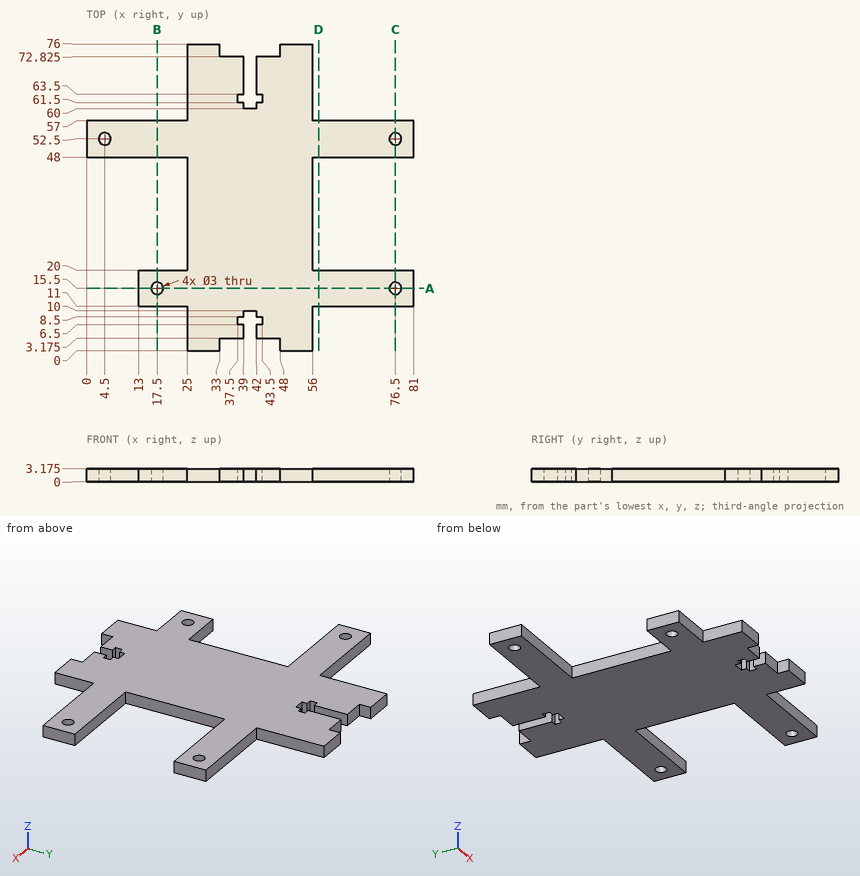
Check sheet for the drawn part. Datum: minimum x, y, z corner. Units: mm. Coordinates: 2 decimals unless noted, no trailing zeros. Loops run counter-clockwise (first coordinate to the right, second up) from the corner with the lowest first, then second, coordinate; pieces in that order, holes last. Notation, with made-up numbers: M 28,-17 L 81,-17 A4 ccw 81,-10 Z; hole C 58.25,28 d1. An arc over 180 degrees is marked long. Answer as a JSON object with one key per item and string values.
1. Depth check by flat-ended pin: P1, Ø0.6, axis at y = 62.5, z = 2.5, coming from the +X side; P2, Ø1.2, axis at y = 9, z = 1.5, coming from the -X side; P3, Ø1, axis at x = 34.5, y = 44, coming from the -Z side; P4, Ø2.5, axis at x = 76.5, y = 15.5, coming from the -Z side. Enter the tip coordinate at first touch or a pass-through.
Outcome:
{"P1": "x = 56", "P2": "x = 25", "P3": "z = 0", "P4": "through"}
2. Sectioned sample at B-B on x = 17.5. Record the cut outline in (y, z) (3 decimals), and give its area (3 significant figures).
Outcome:
{"outline": "M 11,0 L 14,0 L 14,3.175 L 11,3.175 Z; M 17,0 L 20,0 L 20,3.175 L 17,3.175 Z; M 48,0 L 57,0 L 57,3.175 L 48,3.175 Z", "area": "47.6 mm²"}
3. Sectioned sample at D-D on x = 57.5. Record the cut outline in (y, z) (3 decimals), and give its area (4 significant figures).
Outcome:
{"outline": "M 11,0 L 20,0 L 20,3.175 L 11,3.175 Z; M 48,0 L 57,0 L 57,3.175 L 48,3.175 Z", "area": "57.15 mm²"}
4. Scan lines: L1, parallel to Y at x = 76.5, z = 0.85; L2, parallel to Y at x = 24, z = 1.05; L3, parallel to X at y = 70.5, z = 2.9. Record each from-to range of solid material in increasing order. Write a range as from..to.
Outcome:
{"L1": "11..14, 17..20, 48..51, 54..57", "L2": "11..20, 48..57", "L3": "25..39, 42..56"}
5. Sectioned sample at A-A on y = 15.5. Record the cut outline in (x, z) (3 decimals).
Outcome:
{"outline": "M 13,0 L 16,0 L 16,3.175 L 13,3.175 Z; M 19,0 L 75,0 L 75,3.175 L 19,3.175 Z; M 78,0 L 81,0 L 81,3.175 L 78,3.175 Z"}
6. Sectioned sample at C-C on x = 76.5. Record the cut outline in (y, z) (3 decimals).
Outcome:
{"outline": "M 11,0 L 14,0 L 14,3.175 L 11,3.175 Z; M 17,0 L 20,0 L 20,3.175 L 17,3.175 Z; M 48,0 L 51,0 L 51,3.175 L 48,3.175 Z; M 54,0 L 57,0 L 57,3.175 L 54,3.175 Z"}
